from build123d import *

# Parameters (mm, degrees)
BOSS_EXTRUDE1_DEPTH = 66.675
CUT_EXTRUDE1_REACH  = 75.8
CUT_EXTRUDE2_REACH  = 75.8
SKETCH6_W           = 5.842
SKETCH6_H           = 4.878381591
CUT_EXTRUDE4_DEPTH  = 74.800184057


with BuildPart() as part:
    # Sketch1 → Boss-Extrude1 (new body)
    with BuildSketch(Plane(origin=(0, 0, -3683), x_dir=(-1, 0, 0), z_dir=(0, 0, -1))):
        with BuildLine():
            Line((7.945265893, 3.588862728), (-1.198734107, 3.588862728))
            ThreePointArc((-1.198734107, 3.588862728), (-1.647746913, 3.774849922), (-1.833734107, 4.223862728))
            Line((-1.833734107, 4.223862728), (-1.833734107, 5.747862728))
            ThreePointArc((-1.833734107, 5.747862728), (-1.647746913, 6.196875535), (-1.198734107, 6.382862728))
            Line((-1.198734107, 6.382862728), (1.621629442, 6.382862728))
            Line((1.621629442, 6.382862728), (1.621629442, 6.890862686))
            Line((1.621629442, 6.890862686), (-2.214734107, 11.462862728))
            Line((-2.214734107, 11.462862728), (-7.294734107, 11.462862728))
            Line((-7.294734107, 11.462862728), (-11.131097656, 6.890862686))
            Line((-11.131097656, 6.890862686), (-11.131097656, 6.382862728))
            Line((-11.131097656, 6.382862728), (-8.310734107, 6.382862728))
            ThreePointArc((-8.310734107, 6.382862728), (-7.861721301, 6.196875535), (-7.675734107, 5.747862728))
            Line((-7.675734107, 5.747862728), (-7.675734107, 4.223862728))
            ThreePointArc((-7.675734107, 4.223862728), (-7.861721301, 3.774849922), (-8.310734107, 3.588862728))
            Line((-8.310734107, 3.588862728), (-17.454734107, 3.588862728))
            Line((-17.454734107, 3.588862728), (-17.727921752, 3.588862728))
            Line((-17.727921752, 3.588862728), (-17.727921752, 3.858842754))
            Line((-17.727921752, 3.858842754), (-17.728361466, 13.002372481))
            ThreePointArc((-17.728361466, 13.002372481), (-17.542256287, 13.451715967), (-17.092921752, 13.637842754))
            Line((-17.092921752, 13.637842754), (-15.568921752, 13.637842754))
            ThreePointArc((-15.568921752, 13.637842754), (-15.119908946, 13.45185556), (-14.933921752, 13.002842754))
            Line((-14.933921752, 13.002842754), (-14.933921752, 10.182479205))
            Line((-14.933921752, 10.182479205), (-14.425921794, 10.182479205))
            Line((-14.425921794, 10.182479205), (-9.853921752, 14.018842754))
            Line((-9.853921752, 14.018842754), (-9.853921752, 19.098842754))
            Line((-9.853921752, 19.098842754), (-14.425921794, 22.935206303))
            Line((-14.425921794, 22.935206303), (-14.933921752, 22.935206303))
            Line((-14.933921752, 22.935206303), (-14.933921752, 20.114842754))
            ThreePointArc((-14.933921752, 20.114842754), (-15.119908946, 19.665829948), (-15.568921752, 19.479842754))
            Line((-15.568921752, 19.479842754), (-17.092921752, 19.479842754))
            ThreePointArc((-17.092921752, 19.479842754), (-17.542476558, 19.66604812), (-17.728703542, 20.11559397))
            Line((-17.728703542, 20.11559397), (-17.728839138, 22.935206303))
            Line((-17.728839138, 22.935206303), (-21.787214199, 22.935206303))
            Line((-21.787214199, 22.935206303), (-21.791921752, 3.859128788))
            Line((-21.791921752, 3.859128788), (-21.791921752, 3.588862728))
            Line((-21.791921752, 3.588862728), (-21.791921752, -0.475137272))
            Line((-21.791921752, -0.475137272), (-17.727921752, -0.475137272))
            Line((-17.727921752, -0.475137272), (-17.454774021, -0.475137272))
            Line((-17.454774021, -0.475137272), (7.945225979, -0.475137272))
            Line((7.945225979, -0.475137272), (8.215492039, -0.475137272))
            Line((8.215492039, -0.475137272), (8.215492039, 3.588862728))
            Line((8.215492039, 3.588862728), (7.945265893, 3.588862728))
        make_face()
    extrude(amount=BOSS_EXTRUDE1_DEPTH)

    # Sketch2 → Cut-Extrude1 (cut, up to next)
    with BuildSketch(Plane.XY.offset(-3683), mode=Mode.PRIVATE) as cut_extrude1_sk1:
        with BuildLine():
            Line((11.131097656, 6.890862686), (11.131097656, 6.382862728))
            Line((11.131097656, 6.382862728), (8.310734107, 6.382862728))
            ThreePointArc((8.310734107, 6.382862728), (7.861721301, 6.196875535), (7.675734107, 5.747862728))
            Line((7.675734107, 5.747862728), (7.675734107, 11.00880461))
            Line((7.675734107, 11.00880461), (11.131097656, 6.890862686))
        make_face()
    cut_extrude1_tool1 = extrude(cut_extrude1_sk1.sketch, amount=-CUT_EXTRUDE1_REACH, mode=Mode.PRIVATE) & part.part
    # Sketch2 → Cut-Extrude1 (cut, up to next)
    with BuildSketch(Plane.XY.offset(-3683), mode=Mode.PRIVATE) as cut_extrude1_sk2:
        with BuildLine():
            Line((1.833734107, 5.747862728), (1.833734107, 11.00880461))
            Line((1.833734107, 11.00880461), (-1.621629442, 6.890862686))
            Line((-1.621629442, 6.890862686), (-1.621629442, 6.382862728))
            Line((-1.621629442, 6.382862728), (1.198734107, 6.382862728))
            ThreePointArc((1.198734107, 6.382862728), (1.647746913, 6.196875535), (1.833734107, 5.747862728))
        make_face()
    cut_extrude1_tool2 = extrude(cut_extrude1_sk2.sketch, amount=-CUT_EXTRUDE1_REACH, mode=Mode.PRIVATE) & part.part
    add(cut_extrude1_tool1.solids().sort_by_distance((8.930632, 7.925168, -3683))[0], mode=Mode.SUBTRACT)
    add(cut_extrude1_tool2.solids().sort_by_distance((0.578837, 7.925168, -3683))[0], mode=Mode.SUBTRACT)

    # Sketch3 → Cut-Extrude2 (cut, up to next)
    with BuildSketch(Plane.XY.offset(-3683), mode=Mode.PRIVATE) as cut_extrude2_sk1:
        with BuildLine():
            Line((15.568921752, 19.479842754), (10.307979871, 19.479842754))
            Line((10.307979871, 19.479842754), (14.425921794, 22.935206303))
            Line((14.425921794, 22.935206303), (14.933921752, 22.935206303))
            Line((14.933921752, 22.935206303), (14.933921752, 20.114842754))
            ThreePointArc((14.933921752, 20.114842754), (15.119908946, 19.665829948), (15.568921752, 19.479842754))
        make_face()
    cut_extrude2_tool1 = extrude(cut_extrude2_sk1.sketch, amount=-CUT_EXTRUDE2_REACH, mode=Mode.PRIVATE) & part.part
    # Sketch3 → Cut-Extrude2 (cut, up to next)
    with BuildSketch(Plane.XY.offset(-3683), mode=Mode.PRIVATE) as cut_extrude2_sk2:
        with BuildLine():
            Line((10.307979871, 13.637842754), (14.425921794, 10.182479205))
            Line((14.425921794, 10.182479205), (14.933921752, 10.182479205))
            Line((14.933921752, 10.182479205), (14.933921752, 13.002842754))
            ThreePointArc((14.933921752, 13.002842754), (15.119908946, 13.45185556), (15.568921752, 13.637842754))
            Line((15.568921752, 13.637842754), (10.307979871, 13.637842754))
        make_face()
    cut_extrude2_tool2 = extrude(cut_extrude2_sk2.sketch, amount=-CUT_EXTRUDE2_REACH, mode=Mode.PRIVATE) & part.part
    add(cut_extrude2_tool1.solids().sort_by_distance((13.391616, 20.73474, -3683))[0], mode=Mode.SUBTRACT)
    add(cut_extrude2_tool2.solids().sort_by_distance((13.391616, 12.382945, -3683))[0], mode=Mode.SUBTRACT)

    # Sketch6 → Cut-Extrude4 (cut, through all)
    with BuildSketch(Plane(origin=(0, 0, -3749.675), x_dir=(-1, 0, 0), z_dir=(0, 0, -1))):
        with Locations((-4.754734107, 9.374581689)):
            Rectangle(SKETCH6_W, SKETCH6_H)
    extrude(amount=-CUT_EXTRUDE4_DEPTH, mode=Mode.SUBTRACT)


solid = part.part
Could you check a few things on this model? Use its own coordinates, in mm. A direction names the side the tool comes from. Coordinates: 2 decimals unless noted, no trailing zeros. Order: outer loops, then holes, each group sorted by start corner. A loop starts at its lowest first (then second) coordinate and runs counter-clockwise, first axis right, second up.
Q1. Please list where these lines run through material, in increasing order: L1, parallel to X at y = 6.25, z = -3708.5; L2, parallel to Y at x = 11, z = -3727.5; L3, parallel to X at y = 9.5, z = -3737.5.
Q2. Suppose I cut it at A-A on x = 16. Please give me the cut outline in (y, z) (3 decimals).
Q3. Suppose I cut it at D-D on y = 12. Please give me the cut outline in (x, z) (3 decimals), and give its area (3 significant figures).
Q4. Thinking about a two-plate mould opening in Y: for faces 3 (the flat face through (-4, 3.589, -3716)), 4 (the flat face through (13, 3.589, -3716)), 5 (the flat face through (14, 13.638, -3716)), 6 (the flat face through (7.676, 6, -3716)), which applies, released by +Y, released by -Y, zero draft, split by the parting line, or undercut?
Q5. Will these pins go through, and if not, where does the flat tip stop? pin 1 (1.5 mm diameter, centred on y = 17.5, z = -3706, fed in from -X); pin 2 (2 mm diameter, centred on y = 5.5, z = -3717.5, fed in from -X); pin 3 (2 mm diameter, centred on x = 0, z = -3711, fed in from +Y).
Q6. Which directions (+Z, -Z, +X, -X, +Y, -Y) give clear straight access to the entire face, cutting with the end or side of a thin tool? Please do faces 1 (the flat face through (20, 22.935, -3716)), 2 (the flat face through (5, 6.935, -3717)).
Q7. Suppose I cut it at C-C on x = 4. Please give me the cut outline in (y, z) (3 decimals), and give its area (3 significant figures).
Answer:
1. L1: x = 1.83 to 7.68, 17.73 to 21.79
1. L2: y = -0.48 to 3.59, 13.64 to 19.48
1. L3: x = 17.73 to 21.79
2. outline: (-0.475, -3749.675) - (3.589, -3749.675) - (3.589, -3683) - (-0.475, -3683) - close; (13.638, -3749.675) - (19.48, -3749.675) - (19.48, -3683) - (13.638, -3683) - close
3. outline: (17.728, -3749.675) - (21.79, -3749.675) - (21.79, -3683) - (17.728, -3683) - close
3. area: 271 mm2
4. face 3: released by +Y
4. face 4: undercut
4. face 5: undercut
4. face 6: zero draft
5. pin 1: stops at x = 9.85
5. pin 2: stops at x = 1.83
5. pin 3: stops at y = 3.59
6. face 1: +Z, -Z, +X, -X, +Y
6. face 2: +Z, -Z, -X, +Y
7. outline: (-0.475, -3749.675) - (6.935, -3749.675) - (6.935, -3683) - (-0.475, -3683) - close
7. area: 494 mm2
